The model under review builds one solid part; all positions refer to its coordinate system, in mm. Give positions to 0.01 mm unless a question says otherwise; leave off trailing zeros. Order: outer loops, then holes, each group sorted by start corner. A loop starts at its lowest first (then second) coordinate and runs counter-clockwise, first axis right, second up. Notation, with made-up numbers: (30, 13.25) - (86, 13.25) arc R17 cw to (86, 37.25) - close; hole circle Ø2 at (-8, -25.5). An arc over 180 degrees is marked (long way). Use CSV: the item, a comma, the result in double quotes.
Autodesk Inventor part; units mm, degrees
ref_plane "YZ Plane" through (0, 0, 0) normal (1, 0, 0) x (0, 1, 0)
ref_plane "XZ Plane" through (0, 0, 0) normal (0, 1, 0) x (-1, 0, 0)
ref_plane "XY Plane" through (0, 0, 0) normal (0, 0, 1) x (1, 0, 0)
sketch "Sketch1" plane through (0, 0, 0) normal (0, 0, 1) x (1, 0, 0)
  line L0 (-34.925, -22.225) -> (34.925, -22.225)
  line L1 (34.925, -22.225) -> (34.925, 22.225)
  line L2 (34.925, 22.225) -> (-34.925, 22.225)
  line L3 (-34.925, 22.225) -> (-34.925, -22.225)
  line L4 (-34.925, -22.225) -> (34.925, 22.225) construction
  line L5 (34.925, -22.225) -> (-34.925, 22.225) construction
  point P0 (0, 0)
  dimension "d0" = 69.85
  dimension "d1" = 44.45
extrude "Extrusion1" add sketch "Sketch1" along normal blind 4.64
sketch "Sketch2" plane through (0, 0, 4.64) normal (0, 0, 1) x (1, 0, 0)
  line L0 (-34.925, -22.225) -> (34.925, -22.225)
  line L1 (-34.925, 22.225) -> (-34.925, -22.225)
  point P0 (0, 0)
  point P1 (-19.045, 3.175)
  point P2 (19.055, 3.175)
  dimension "d4" = 25.4
  dimension "d5" = 15.88
  dimension "d6" = 38.1
hole "Hole1" at (-19.045, 3.175, 4.64) at (19.055, 3.175, 4.64) direction (0, 0, -1) diameter 4.917 depth 15 tip angle 118 countersink diameter 12 countersink angle 90
properties part number "plaka"
Item 1: Clearance check with flat-ended pins moving along their axes: pin 1 (8 mm diameter, centred on x = 19.055, y = 3.175, fed in from +Z); pin 2 (6.5 mm diameter, centred on x = -19.045, y = 3.175, fed in from +Z). State where each tip first meets the part, or that it passes through.
Results list:
pin 1,"stops at z = 2.64"
pin 2,"stops at z = 1.89"
Item 2: Mouldability with a two-part tool opening along X and no side actions: class faces 1 (the face through (0, -22.225, 2)), 2 (the face through (-21.66, 3.76, 1.32)), 3 (the face through (34.925, 0, 2)), 4 (the face through (-34.925, 0, 2)) as pulls with the +X half, pulls with the -X half, needs draft (parallel to the pull), parting line crosses it, or undercut.
Results list:
face 1,"needs draft"
face 2,"undercut"
face 3,"pulls with the +X half"
face 4,"pulls with the -X half"
Item 3: Wall thickness on L1, parallel to X at y = 4, z = 3.25 (3 decimals); L2, parallel to X at y = 5, z = 2.8 (3 decimals); L3, parallel to Y at x = 17, z = 0.7 (3 decimals): over which ranges is each line inside the solid? List them lowest first.
Results list:
L1,"x = -34.925 to -23.581, -14.509 to 14.519, 23.591 to 34.925"
L2,"x = -34.925 to -22.783, -15.307 to 15.317, 22.793 to 34.925"
L3,"y = -22.225 to 1.825, 4.525 to 22.225"
Item 4: Take a section at A-A, the plane z = 3.35. Give the boundary of the cut face in (x, y) (3 decimals), and give its area (3 significant figures).
Results list:
outline,"(-34.925, -22.225) - (34.925, -22.225) - (34.925, 22.225) - (-34.925, 22.225) - close; hole circle Ø9.42 at (-19.045, 3.175); hole circle Ø9.42 at (19.055, 3.175)"
area,"2,970 mm2"
